from build123d import *

# Parameters (mm, degrees)
SKETCH1_W               = 80
SKETCH1_H               = 60
BOSS_EXTRUDE1_DEPTH     = 5
SKETCH2_W               = 50.2
SKETCH2_H               = 44.2
SKETCH2_W_2             = 30.2
SKETCH2_H_2             = 24.2
BOSS_EXTRUDE2_DEPTH     = 25
CUT_EXTRUDE1_DEPTH      = 87.810195254
CUT_EXTRUDE1_DEPTH_BACK = 87.810195254
SKETCH3_W               = 10
SKETCH3_H               = 15
SKETCH4_W               = 50.2
SKETCH4_H               = 7.9
BOSS_EXTRUDE3_DEPTH     = 25
CHAMFER1_SIZE           = 7.7
SKETCH5_W               = 14.9
SKETCH5_H               = 25
BOSS_EXTRUDE4_DEPTH     = 5
SKETCH6_R               = 2.25
CUT_EXTRUDE3_DEPTH      = 5
CUT_EXTRUDE4_DEPTH      = 107.066017178
CUT_EXTRUDE4_DEPTH_BACK = 107.066017178
SKETCH7_R               = 2.15


with BuildPart() as part:
    # Sketch1 → Boss-Extrude1 (new body)
    with BuildSketch(Plane.XY):
        with Locations((40, 30)):
            Rectangle(SKETCH1_W, SKETCH1_H)
    extrude(amount=BOSS_EXTRUDE1_DEPTH)

    # Sketch2 → Boss-Extrude2 (add)
    with BuildSketch(Plane.XY.offset(5)):
        with Locations((40, 30)):
            Rectangle(SKETCH2_W, SKETCH2_H)
        with Locations((40, 30)):
            Rectangle(SKETCH2_W_2, SKETCH2_H_2, mode=Mode.SUBTRACT)
    extrude(amount=BOSS_EXTRUDE2_DEPTH)

    # Sketch3 → Cut-Extrude1 (cut, two sides: drawn at the far end of the back side and taken through both)
    with BuildSketch(Plane.ZY.offset(-55.1).offset(-CUT_EXTRUDE1_DEPTH_BACK)):
        with Locations((20, 44.6)):
            Rectangle(SKETCH3_W, SKETCH3_H)
    extrude(amount=CUT_EXTRUDE1_DEPTH + CUT_EXTRUDE1_DEPTH_BACK, mode=Mode.SUBTRACT)

    # Sketch4 → Boss-Extrude3 (add)
    with BuildSketch(Plane.XY.offset(5)):
        with Locations((40, 56.05)):
            Rectangle(SKETCH4_W, SKETCH4_H)
    extrude(amount=BOSS_EXTRUDE3_DEPTH)

    # Chamfer1
    chamfer1_edges = [part.edges().sort_by_distance(p)[0] for p in [
        (40, 42.1, 5),
    ]]
    chamfer(chamfer1_edges, length=CHAMFER1_SIZE)

    # Sketch5 → Boss-Extrude4 (add)
    with BuildSketch(Plane(origin=(0, 60, 0), x_dir=(1, 0, 0), z_dir=(0, 1, 0))):
        with Locations((7.45, -17.5)):
            Rectangle(SKETCH5_W, SKETCH5_H)
        Polygon((80, -5), (80, 0), (0, 0), (0, -5), (14.9, -5), (14.9, -30), (65.1, -30), (65.1, -5), align=None)
        with Locations((72.55, -17.5)):
            Rectangle(SKETCH5_W, SKETCH5_H)
    extrude(amount=BOSS_EXTRUDE4_DEPTH)

    # Sketch6 → Cut-Extrude3 (cut)
    with BuildSketch(Plane.XZ.offset(-60)):
        with Locations(Location((7, 20, 0), (0, 0, 270))):
            Circle(SKETCH6_R)
    cut_extrude3 = extrude(amount=-CUT_EXTRUDE3_DEPTH, mode=Mode.SUBTRACT)

    # Mirror1: Cut-Extrude3 across plane
    add(cut_extrude3.mirror(Plane.ZY.offset(-40)), mode=Mode.SUBTRACT)

    # Sketch7 → Cut-Extrude4 (cut, two sides: drawn at the far end of the back side and taken through both)
    with BuildSketch(Plane.XY.offset(5).offset(-CUT_EXTRUDE4_DEPTH_BACK)):
        with Locations((8, 30)):
            Circle(SKETCH7_R)
        with Locations(Location((72, 30, 0), (0, 0, 180))):
            Circle(SKETCH7_R)
    extrude(amount=CUT_EXTRUDE4_DEPTH + CUT_EXTRUDE4_DEPTH_BACK, mode=Mode.SUBTRACT)


solid = part.part
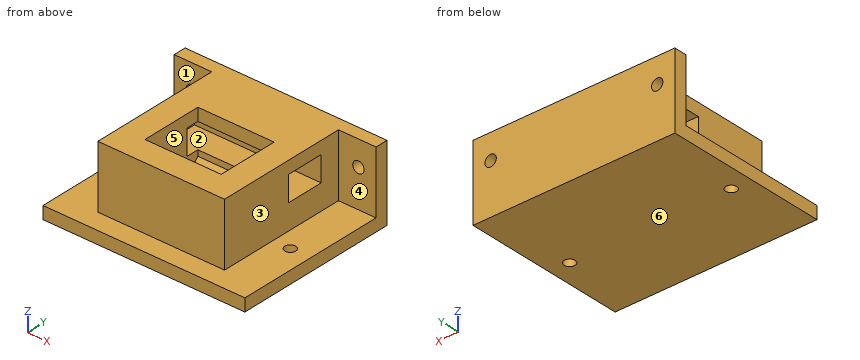
Build history of the part. All positions in model axes, mm. Face numbers are marked on the shaded views. A direction names the side the tool comes from. Coordinates: 2 decimals unless noted, no trailing zeros. Order: outer loops, then holes, each group sorted by start corner. A loop starts at its lowest first (then second) coordinate and runs counter-clockwise, first axis right, second up. Notation, with made-up numbers: (46.5, 21) - (80.5, 21) arc R34 ccw to (80.5, 53) - close; hole circle Ø5 at (-29, 79.5). An arc over 180 degrees is marked (long way). Write item = value, one per line. Start each with the question number.
1) Flat gauge pins, fed straight in: pin 1 Ø6 at (x, z) = (19, 25) entering from -Y; pin 2 Ø7 at (x, y) = (8, 30) entering from +Z; pin 3 Ø1 at (y, z) = (33, 18) entering from -X; pin 4 Ø18 at (x, y) = (54.5, 33.5) entering from +Z. Where does each tip first touch, or does it go through?
2) 3-axis set-ups, long thin cutter, end or side, ignore diameter. For the marked faces 1, 2 and 3: which of +Z, -Z, +X, -X, +Y, -Y reach the whole face in a straight line?
3) Saw through at B-B on z = 20. Write the cut outline in (x, y), then the cut area to 3 significant figures.
4) Saw through at D-D on z = 8.5. Write the cut outline in (x, y).
5) Saw through at C-C on x = 73. Write the cut outline in (y, z), then the cut area to 3 significant figures.
6) Two-plate mould, pull along Y, no slides. Class the marked faces 4, 5 and 6: pulls with the +Y half, pulls with the -Y half, needs draft (parallel to the pull), parting line crosses it, or undercut.
7) Saw through at A-A on y = 45. Write the cut outline in (x, z).
8) Wall check: line 1 along X through (y, z) = (63.1, 20); line 2 along Z through (x, y) = (73, 63.65); line 3 along Y through (x, z) = (72, 2.9). Give the ranges that are in metal, low to high. Write a range as from..to.
From the geometry:
q1.pin_1 = 7.9
q1.pin_2 = 5
q1.pin_3 = 14.9
q1.pin_4 = 30
q2.face_1 = +Z, -X, -Y
q2.face_2 = +X, -X
q2.face_3 = +Z, +X, -Y
q3.outline = (0, 60) - (4.75, 60) - (4.75, 65) - (0, 65) - close; (9.25, 60) - (14.9, 60) - (14.9, 52.1) - (65.1, 52.1) - (65.1, 60) - (70.75, 60) - (70.75, 65) - (9.25, 65) - close; (14.9, 7.9) - (65.1, 7.9) - (65.1, 37.1) - (55.1, 37.1) - (55.1, 17.9) - (24.9, 17.9) - (24.9, 37.1) - (14.9, 37.1) - close; (75.25, 60) - (80, 60) - (80, 65) - (75.25, 65) - close
q3.area = 1,640 mm^2
q4.outline = (0, 60) - (14.9, 60) - (14.9, 7.9) - (65.1, 7.9) - (65.1, 60) - (80, 60) - (80, 65) - (0, 65) - close; hole (24.9, 17.9) - (55.1, 17.9) - (55.1, 37.9) - (24.9, 37.9) - close
q5.outline = (0, 0) - (28.1, 0) - (28.1, 5) - (0, 5) - close; (31.9, 0) - (65, 0) - (65, 17.75) - (60, 17.75) - (60, 5) - (31.9, 5) - close; (60, 22.25) - (65, 22.25) - (65, 30) - (60, 30) - close
q5.area = 408 mm^2
q6.face_4 = pulls with the -Y half
q6.face_5 = undercut
q6.face_6 = needs draft
q7.outline = (0, 0) - (80, 0) - (80, 5) - (65.1, 5) - (65.1, 15) - (14.9, 15) - (14.9, 5) - (0, 5) - close; (14.9, 25) - (65.1, 25) - (65.1, 30) - (14.9, 30) - close
q8.line_1 = 0..4.75, 9.25..70.75, 75.25..80
q8.line_2 = 0..17.75, 22.25..30
q8.line_3 = 0..27.85, 32.15..65
